CAD build for the part. Positions are in the model's coordinates, mm. Face numbers are marked on the shaded views. A direction names the side the tool comes from. Round coordinates to 2 decimals unless told otherwise and drop trailing zeros. Order: outer loops, then holes, each group sorted by start corner. A loop starts at its lowest first (then second) coordinate and runs counter-clockwise, first axis right, second up. Notation, with made-up numbers: (-27.5, -22) -> (-20.5, -22) arc R18 cw to (-20.5, -10) -> close; hole circle Ø2 at (16, 76.25). An arc over 180 degrees is marked (long way). Return JSON: item names as keys, results as strings. Group by question number.
Q1. Which spindle directions (+Z, -Z, +X, -X, +Y, -Y) get a long thin tool onto all of the face, cutting with end or side? Do the marked faces 1 and 2. Say none if no direction does.
Q2. Cut at D-D (y = 3.2). Write the cut outline in (x, z), then the cut area to 3 significant figures.
Q3. Cut at A-A (z = 0). Write the cut outline in (x, y), then the cut area to 3 significant figures.
Q4. Flat gauge pins, fed straight in: pin 1 (2 mm diameter, centred on y = 2.5, z = 7, fed in from -X); pin 2 (5 mm diameter, centred on x = 7.15, z = 0, fed in from +Y); pin 3 (2.5 mm diameter, centred on x = -7.15, z = 0, fed in from -Y). Where does each tip first touch, or does it go through?
Q5. Cut at C-C (z = -7.15). Write the cut outline in (x, y), then the cut area to 3 significant figures.
Q6. Probe line 1 along X through (y, z) = (0.6, 0); line 2 along Y through (x, z) = (1, 6); line 3 along Z through (x, y) = (-8.25, 2.25). List the from-to ranges inside material, lowest first.
Q7. Mould opens along X. For the marked faces 3, 4 and 5 say: +X half, -X half, draft (parallel to the pull), parting line (faces both ways), or undercut.
Q8. Cut at B-B (x = -7.15). Write the cut outline in (y, z).
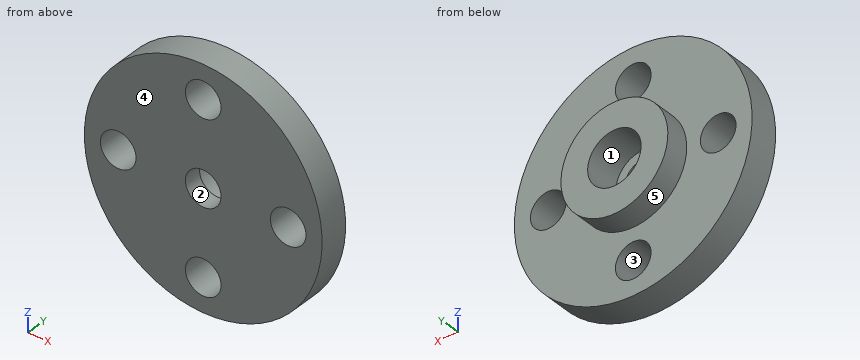
from build123d import *

# Parameters (mm, degrees)
SKETCH1_R           = 10
SKETCH1_R_2         = 1.5
BOSS_EXTRUDE1_DEPTH = 2.5
SKETCH2_R           = 4.5
BOSS_EXTRUDE2_DEPTH = 2
SKETCH3_R           = 2.25
CUT_EXTRUDE1_DEPTH  = 3


with BuildPart() as part:
    # Sketch1 → Boss-Extrude1 (new body)
    with BuildSketch(Plane(origin=(0, 0, 0), x_dir=(1, 0, 0), z_dir=(0, 1, 0))):
        with Locations(Location((0, 0, 0), (0, 0, 270))):
            Circle(SKETCH1_R)
        with Locations(Location((0, 0, 0), (0, 0, 270))):
            Circle(SKETCH1_R_2, mode=Mode.SUBTRACT)
        with Locations(Location((0, 7.15, 0), (0, 0, 270))):
            Circle(SKETCH1_R_2, mode=Mode.SUBTRACT)
        with Locations(Location((7.15, 0, 0), (0, 0, 270))):
            Circle(SKETCH1_R_2, mode=Mode.SUBTRACT)
        with Locations(Location((0, -7.15, 0), (0, 0, 270))):
            Circle(SKETCH1_R_2, mode=Mode.SUBTRACT)
        with Locations(Location((-7.15, 0, 0), (0, 0, 270))):
            Circle(SKETCH1_R_2, mode=Mode.SUBTRACT)
    extrude(amount=BOSS_EXTRUDE1_DEPTH)

    # Sketch2 → Boss-Extrude2 (add)
    with BuildSketch(Plane(origin=(0, 2.5, 0), x_dir=(1, 0, 0), z_dir=(0, 1, 0))):
        with Locations(Location((0, 0, 0), (0, 0, 270))):
            Circle(SKETCH2_R)
    extrude(amount=BOSS_EXTRUDE2_DEPTH)

    # Sketch3 → Cut-Extrude1 (cut)
    with BuildSketch(Plane(origin=(0, 4.5, 0), x_dir=(1, 0, 0), z_dir=(0, 1, 0))):
        with Locations(Location((0, 0, 0), (0, 0, 270))):
            Circle(SKETCH3_R)
    extrude(amount=-CUT_EXTRUDE1_DEPTH, mode=Mode.SUBTRACT)


solid = part.part
Solution:
{
 "1": {"face 1": "+Y", "face 2": "+Y, -Y"},
 "2": {"outline": "circle Ø9 at (0, 0); hole circle Ø4.5 at (0, 0)", "area": "47.7 mm²"},
 "3": {"outline": "(-10, 0) -> (-8.65, 0) -> (-8.65, 2.5) -> (-10, 2.5) -> close; (-5.65, 0) -> (-1.5, 0) -> (-1.5, 1.5) -> (-2.25, 1.5) -> (-2.25, 4.5) -> (-4.5, 4.5) -> (-4.5, 2.5) -> (-5.65, 2.5) -> close; (1.5, 0) -> (5.65, 0) -> (5.65, 2.5) -> (4.5, 2.5) -> (4.5, 4.5) -> (2.25, 4.5) -> (2.25, 1.5) -> (1.5, 1.5) -> close; (8.65, 0) -> (10, 0) -> (10, 2.5) -> (8.65, 2.5) -> close", "area": "35.0 mm²"},
 "4": {"pin 1": "stops at x = -8", "pin 2": "stops at y = 2.5", "pin 3": "passes through"},
 "5": {"outline": "(-6.99, 0) -> (-1.5, 0) -> (-1.5, 2.5) -> (-6.99, 2.5) -> close; (1.5, 0) -> (6.99, 0) -> (6.99, 2.5) -> (1.5, 2.5) -> close", "area": "27.5 mm²"},
 "6": {"line 1": "x = -10 to -8.65, -5.65 to -1.5, 1.5 to 5.65, 8.65 to 10", "line 2": "y = 0 to 2.5", "line 3": "z = -5.65 to -1.02, 1.02 to 5.65"},
 "7": {"face 3": "undercut", "face 4": "draft", "face 5": "parting line"},
 "8": {"outline": "(0, -6.99) -> (2.5, -6.99) -> (2.5, -1.5) -> (0, -1.5) -> close; (0, 1.5) -> (2.5, 1.5) -> (2.5, 6.99) -> (0, 6.99) -> close"}
}
